Part model, mm, in its own coordinate system. A direction names the side the tool comes from. Round coordinates to 2 decimals unless told otherwise and drop trailing zeros. Loops run counter-clockwise (first coordinate to the right, second up) from the corner with the lowest first, then second, coordinate; pieces in that order, holes last.
from build123d import *

# Parameters (mm, degrees)
ESQUISSE1_R        = 4
ESQUISSE1_R_2      = 5
BOSS_EXTRU_1_DEPTH = 10


with BuildPart() as part:
    # Esquisse1 → Boss.-Extru.1 (new body)
    with BuildSketch(Plane.XY):
        Polygon((-70, 40), (-70, 10), (-70, -10), (70, -10), (70, 10), (70, 40), (50, 40), (50, 10), (-50, 10), (-50, 40), align=None)
        with Locations((-60, 0)):
            Circle(ESQUISSE1_R, mode=Mode.SUBTRACT)
        Circle(ESQUISSE1_R_2, mode=Mode.SUBTRACT)
        with Locations((60, 0)):
            Circle(ESQUISSE1_R, mode=Mode.SUBTRACT)
        Polygon((-70, 40), (-70, 10), (-70, -10), (70, -10), (70, 10), (70, 40), (50, 40), (50, 10), (-50, 10), (-50, 40), align=None)
        with Locations((-60, 0)):
            Circle(ESQUISSE1_R, mode=Mode.SUBTRACT)
        Circle(ESQUISSE1_R_2, mode=Mode.SUBTRACT)
        with Locations((60, 0)):
            Circle(ESQUISSE1_R, mode=Mode.SUBTRACT)
        Polygon((-70, 40), (-70, 10), (-70, -10), (70, -10), (70, 10), (70, 40), (50, 40), (50, 10), (-50, 10), (-50, 40), align=None)
        with Locations((-60, 0)):
            Circle(ESQUISSE1_R, mode=Mode.SUBTRACT)
        Circle(ESQUISSE1_R_2, mode=Mode.SUBTRACT)
        with Locations((60, 0)):
            Circle(ESQUISSE1_R, mode=Mode.SUBTRACT)
    extrude(amount=BOSS_EXTRU_1_DEPTH)


solid = part.part
1) Slice it at B-B, the plane x = 0. Give the cut face in (y, z), then the cut area to 3 significant figures.
Values:
outline: (-10, 0) - (-5, 0) - (-5, 10) - (-10, 10) - close; (5, 0) - (10, 0) - (10, 10) - (5, 10) - close
area: 100 mm2
2) Slice it at D-D, the plane z = 5.25. Give the cut face in (x, y).
Values:
outline: (-70, -10) - (70, -10) - (70, 40) - (50, 40) - (50, 10) - (-50, 10) - (-50, 40) - (-70, 40) - close; hole circle Ø8 at (-60, 0); hole circle Ø10 at (0, 0); hole circle Ø8 at (60, 0)
3) Mould opens along X. For faces 1 (the face through (-1, 9.8, 0)), 2 (the face through (1, 10, 5)), 3 (the face through (-70, 15, 5)) say: released by +X, released by -X, zero draft, split by the parting line, or undercut.
Values:
face 1: zero draft
face 2: undercut
face 3: released by -X
4) Slice it at C-C, the plane y = 28. Give the cut face in (x, z), then the cut area to 3 significant figures.
Values:
outline: (-70, 0) - (-50, 0) - (-50, 10) - (-70, 10) - close; (50, 0) - (70, 0) - (70, 10) - (50, 10) - close
area: 400 mm2
5) Tool access for faces 4 (the face through (50, 25, 5)), 5 (the face through (-1, -10, 5)): list every direction of +Z, -Z, +X, -X, +Y, -Y with a clear straight run to the whole face (end or side of a thin tool).
Values:
face 4: +Z, -Z, +Y
face 5: +Z, -Z, +X, -X, -Y
6) Drop a flat-ended pin along its axis: pin 1 Ø6 at (x, y) = (-43, -1) entering from -Z. Give the stop position or say it passes through.
Values:
pin 1: stops at z = 0
7) Wall check: line 1 along X through (y, z) = (14.5, 0.75); line 2 along Y through (x, z) = (0, 3.75); line 3 along Y through (x, z) = (-60, 6). Give the ranges that are in metal, low to high.
Values:
line 1: x = -70 to -50, 50 to 70
line 2: y = -10 to -5, 5 to 10
line 3: y = -10 to -4, 4 to 40
8) Slice it at A-A, the plane y = 0. Give the cut face in (x, z).
Values:
outline: (-70, 0) - (-64, 0) - (-64, 10) - (-70, 10) - close; (-56, 0) - (-5, 0) - (-5, 10) - (-56, 10) - close; (5, 0) - (56, 0) - (56, 10) - (5, 10) - close; (64, 0) - (70, 0) - (70, 10) - (64, 10) - close
